Geometry: see drawing. Coordinates: mm, zero at the bounding-box minimum. A direction names the side the tool comes from. Give positions to 0.01 mm unless a question says otherwise; leave off trailing zeros. Loops run counter-clockwise (first coordinate to the right, second up) from the corner with the lowest first, then second, coordinate; pieces in that order, holes last. Notation, with made-up numbers: M 62.25,13 L 113.25,13 A28 ccw 113.25,44 Z; hole C 60.25,72 d9. An arc over 180 degrees is marked long. Put each result on its own line as item: value.
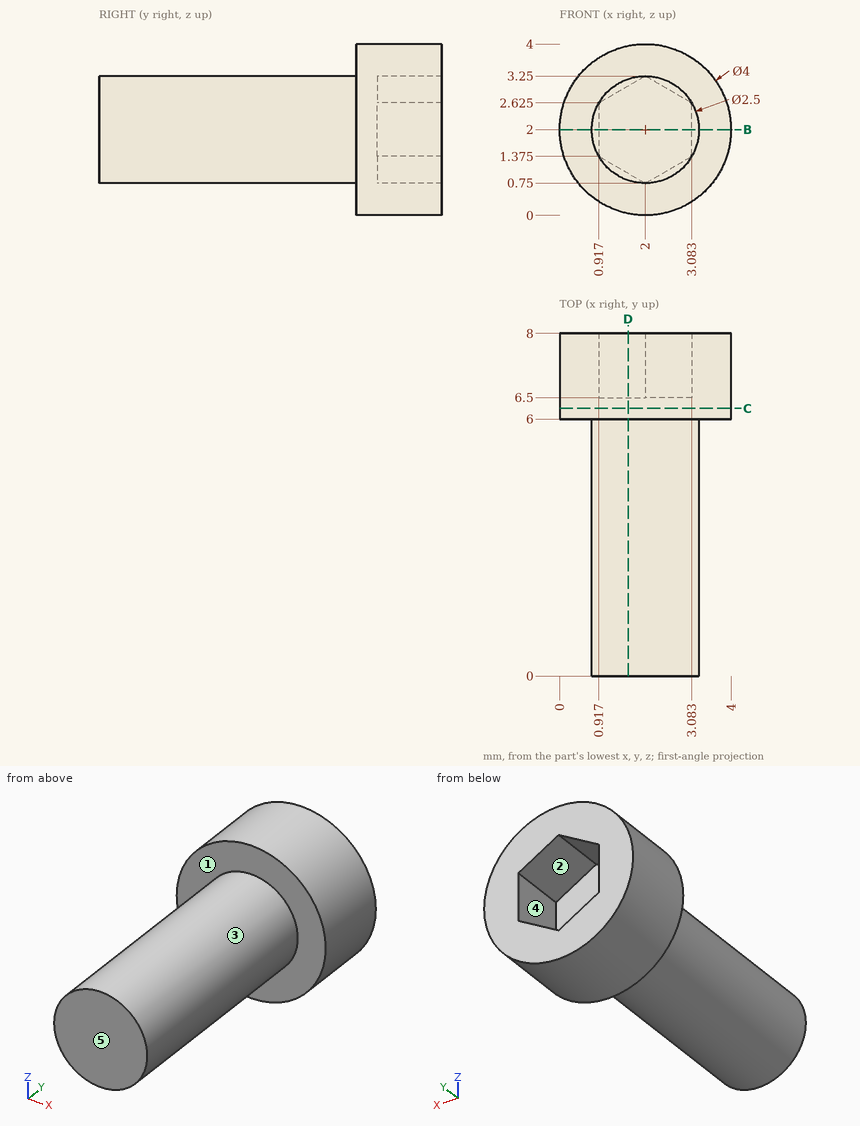
Item 1: Pin query (flat end, axial travel): pin 1 Ø1 at (y, z) = (6, 3) entering from -X; pin 2 Ø1 at (x, z) = (2.5, 2) entering from +Y. Return the tip coordinate at first contact, or that it passes through.
Output values:
pin 1: x = 0.06
pin 2: y = 6.5
Item 2: Set-up query: the marked faces 4 and 5. Return all of +Z, -Z, +X, -X, +Y, -Y with unobstructed straight access to the full face (end or side cutting, diameter ignored); none if empty.
Output values:
face 4: +Y
face 5: +Z, -Z, +X, -X, -Y
Item 3: Section D-D on x = 1.6. Output: boundary loops of the cut face in (y, z) (1 decimal), then the cut area to 3 significant figures.
Output values:
outline: M 0,0.8 L 6,0.8 L 6,0 L 8,0 L 8,1 L 6.5,1 L 6.5,3 L 8,3 L 8,4 L 6,4 L 6,3.2 L 0,3.2 Z
area: 19.0 mm²
Item 4: Section C-C on y = 6.25. Output: boundary loops of the cut face in (x, z), then the cut area to 3 significant figures.
Output values:
outline: C 2,2 d4
area: 12.6 mm²
Item 5: Line query: probe 1 along Y at (x, z) = (3, 2.85); probe 2 along X at (y, z) = (7.75, 2.55); probe 3 along Y at (x, z) = (1, 1.8). Output: solid intervals per line, ascending. Write a range as [from, to].
Output values:
probe 1: [6, 8]
probe 2: [0.08, 0.92], [3.08, 3.92]
probe 3: [0, 6.5]
Item 6: Section B-B on z = 2. Output: boundary loops of the cut face in (x, y).
Output values:
outline: M 0,6 L 0.75,6 L 0.75,0 L 3.25,0 L 3.25,6 L 4,6 L 4,8 L 3.08,8 L 3.08,6.5 L 0.92,6.5 L 0.92,8 L 0,8 Z
Item 7: Mould query, pull axis Z, two halves, no side actions, for the marked faces 1, 2 and 3. Classes: pulls with the +Z half, pulls with the -Z half, needs draft (parallel to the pull), parting line crosses it, or undercut.
Output values:
face 1: needs draft
face 2: undercut
face 3: parting line crosses it
